Verification items for this drawing (mm, ordinates from the low corner). A direction names the side the tool comes from. Coordinates: 2 decimals unless noted, no trailing zeros. Order: outer loops, then holes, each group sorted by start corner. A loop starts at its lowest first (then second) coordinate and runs counter-clockwise, first axis right, second up. Notation, with made-up numbers: M -7.75,54 L 0.25,54 A19 ccw 0.25,71 Z; hole C 26.5,66 d6. An arc over 180 degrees is marked long. Write item = value, one per line.
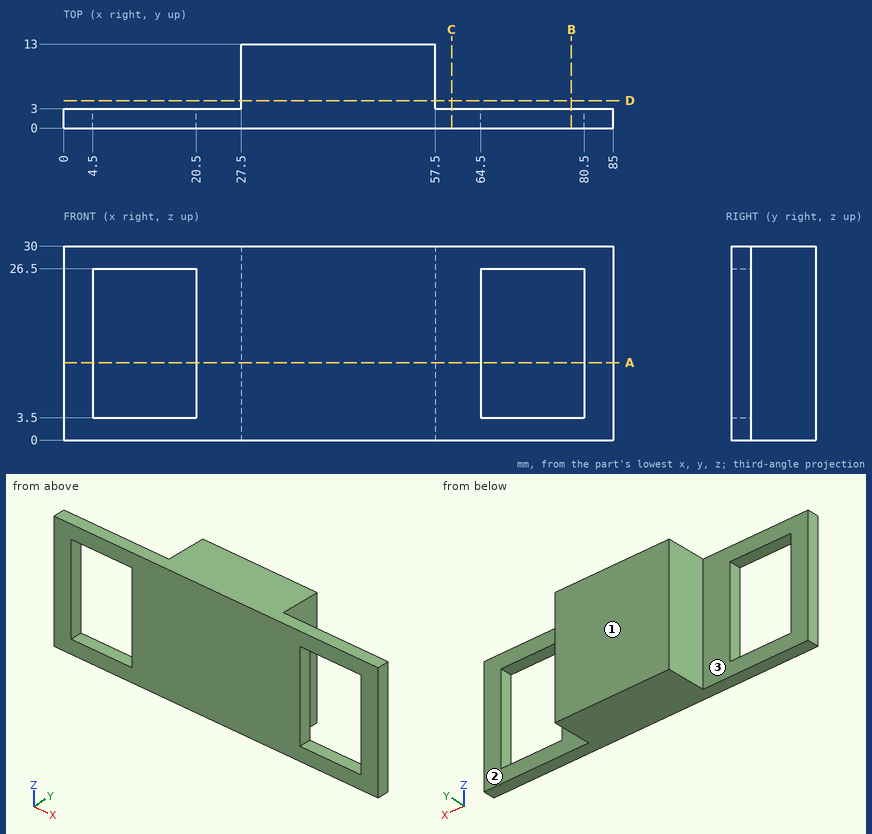
Item 1: Gauge pin test, flat ends, axial feed: pin 1 (1.5 mm diameter, centred on x = 58, y = 3, fed in from -Z); pin 2 (6 mm diameter, centred on y = 8.5, z = 17, fed in from +X). Record the tip position at first contact, or that the pin passes through.
Report:
pin_1 = 0
pin_2 = 57.5
Item 2: Sectioned sample at B-B, the plane x = 78.5. Enter the section's corners in (y, z).
Report:
outline = M 0,0 L 3,0 L 3,3.5 L 0,3.5 Z; M 0,26.5 L 3,26.5 L 3,30 L 0,30 Z
Item 3: Tool access check on the marked faces 1, 2 and 3. Record the directions out of +Z, -Z, +X, -X, +Y, -Y that give a thin tool (end or side, any length) a straight path to the whole face; none if there is none.
Report:
face_1 = +Z, -Z, +X, -X, +Y
face_2 = +Z, -Z, +X, +Y
face_3 = +Z, -Z, -X, +Y
Item 4: Scan lines: L1, parallel to X at y = 2.25, z = 22.25; L2, parallel to X at y = 12.75, z = 24; L3, parallel to Y at x = 4, z = 22. Record each from-to range of solid material in increasing order. Write a range as from..to.
Report:
L1 = 0..4.5, 20.5..64.5, 80.5..85
L2 = 27.5..57.5
L3 = 0..3
Item 5: Sectioned sample at C-C, the plane x = 60. Enter the section's corners in (y, z), then the cut area to 3 significant figures.
Report:
outline = M 0,0 L 3,0 L 3,30 L 0,30 Z
area = 90.0 mm^2
Item 6: Sectioned sample at A-A, the plane z = 12. Enter the section's corners in (x, y), then the cut area to 3 significant figures.
Report:
outline = M 0,0 L 4.5,0 L 4.5,3 L 0,3 Z; M 20.5,0 L 64.5,0 L 64.5,3 L 57.5,3 L 57.5,13 L 27.5,13 L 27.5,3 L 20.5,3 Z; M 80.5,0 L 85,0 L 85,3 L 80.5,3 Z
area = 459 mm^2
Item 7: Sectioned sample at D-D, the plane y = 4.25. Enter the section's corners in (x, z).
Report:
outline = M 27.5,0 L 57.5,0 L 57.5,30 L 27.5,30 Z
